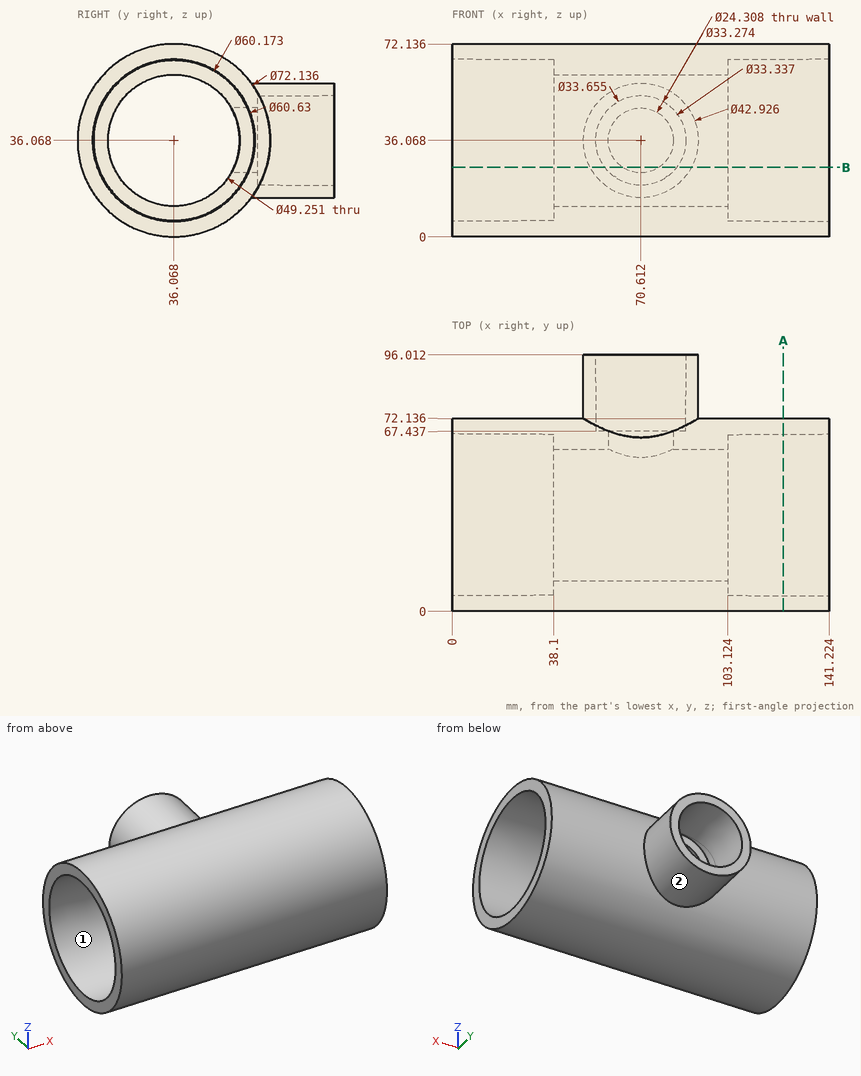
Drawing for the job (mm, zero at the part's lowest x, y, z). Give positions to 0.01 mm unless a question says otherwise; leave off trailing zeros. Order: outer loops, then holes, each group sorted by start corner. A loop starts at its lowest first (then second) coordinate and runs counter-clockwise, first axis right, second up. Notation, with made-up numbers: (-39, 11) - (7, 11) arc R24 ccw to (7, 26) - close; hole circle Ø3 at (12.25, 6.5). An arc over 180 degrees is marked (long way). Use one line per item in the form item = value.
Item 1: Two-plate mould, pull along Z, no slides. Class the marked faces 1 and 2: released by +Z, released by -Z, zero draft, split by the parting line, or undercut.
Solution:
face_1 = undercut
face_2 = split by the parting line
Item 2: Slice it at B-B on z = 26. Count the separate pieces of the cut face and the enclosed holes in it.
Solution:
separate_pieces = 3
enclosed_holes = 0
Item 3: Slice it at A-A on x = 124. Give the cut face in (y, z).
Solution:
outline = circle Ø72.14 at (36.07, 36.07); hole circle Ø60.42 at (36.07, 36.07)
Item 4: Pin check, flat tips, straight feed: pin 1 Ø1 at (x, y) = (77.5, 15) entering from +Z; pin 2 Ø6 at (y, z) = (16, 19.5) entering from -X; pin 3 Ø5 at (x, z) = (110, 18.5) entering from -Y. Stop position of each tip, or through.
Solution:
pin_1 = 65.7
pin_2 = 38.1
pin_3 = 3.3
Item 5: Probe probe 1 along Y at (x, z) = (51, 36.5); probe 2 along X at (y, z) = (85.5, 36) (1 decimal); probe 3 along X at (y, z) = (42, 10.5). List the from-to ranges inside material, lowest first. Write a range as from..to.
Solution:
probe_1 = 0..11.45, 60.69..96.01
probe_2 = 49.1..53.9, 87.4..92.1
probe_3 = 38.1..103.12
